```python
from build123d import *

# Parameters (mm, degrees)
F0_W     = 13
F0_H     = 6
F1_DEPTH = 17
F2_W     = 13.75
F2_H     = 6.75
F2_W_2   = 13
F2_H_2   = 6
F3_DEPTH = 0.5
F4_W     = 12.25
F4_H     = 5.25
F5_DEPTH = 16.5


with BuildPart() as f1:
    # F0 (on Top) → F1 (new body)
    with BuildSketch(Plane.XY):
        Rectangle(F0_W, F0_H)
    extrude(amount=F1_DEPTH)

    # F2 (on face) → F3 (join)
    with BuildSketch(Plane.XY.offset(17)):
        Rectangle(F2_W, F2_H)
        Rectangle(F2_W_2, F2_H_2, mode=Mode.SUBTRACT)
        Rectangle(F2_W_2, F2_H_2)
    extrude(amount=-F3_DEPTH)

    # F4 (on face) → F5 (cut, through all)
    with BuildSketch(Plane.XY.offset(17)):
        Rectangle(F4_W, F4_H)
    extrude(amount=-F5_DEPTH, mode=Mode.SUBTRACT)


solid = f1.part
```
The model under review builds one solid part; all positions refer to its coordinate system, in mm. A direction names the side the tool comes from. Coordinates: 2 decimals unless noted, no trailing zeros. Write each loop counter-clockwise with the first axis right and the second up, starting at its lowest first coordinate (ties: lowest second). Pieces come first, ordered by that corner, then holes.
1) To check wall thickness, follow probe 1 along Y at (x, z) = (2, 12.25) (3 decimals); probe 2 along X at (y, z) = (0.75, 12) (3 decimals); probe 3 along Z at (x, y) = (1.5, 1.75). State the ranges of each line that lie inside material, in increasing order.
2) The part is to be moulded in two halves that separate along Y. For faces 6 (the face through (0, -3, 8)), 7 (the face through (0, 2.625, 9)), 8 (the face through (-6.5, 0, 8)), say which applies: pulls with the +Y half, pulls with the -Y half, needs draft (parallel to the pull), parting line crosses it, or undercut.
3) Clearance check with flat-ended pins moving along their axes: pin 1 Ø3 at (x, z) = (-1, 3.5) entering from -Y; pin 2 Ø1.6 at (y, z) = (-1, 5.5) entering from +X; pin 3 Ø4 at (x, y) = (-1.5, 0.5) entering from +Z. State where each tip first meets the part, or that it passes through.
4) We need section B-B on z = 9.5. State the section outline as (x, y) points (3 decimals), then the cut area to 3 significant figures.
5) Machinability: for faces 1 (the face through (0, 0, 0)), 2 (the face through (0, 3, 8)), 3 (the face through (6.125, 0, 9)), 4 (the face through (6.5, 0, 8)), 5 (the face through (-1, -3, 17)), which of the approach directions +Z, -Z, +X, -X, +Y, -Y give a long, thin tool a straight path to every point of the face, cutting with its end or side? Answer none if there is none.
6) We need section A-A on y = -2.25. State the section outline as (x, z) points (3 decimals).
7) We need section C-C on x = -2. State the section outline as (y, z) points (3 decimals).
Answer list:
1. probe 1: y = -3 to -2.625, 2.625 to 3
1. probe 2: x = -6.5 to -6.125, 6.125 to 6.5
1. probe 3: z = 0 to 0.5
2. face 6: pulls with the -Y half
2. face 7: undercut
2. face 8: needs draft
3. pin 1: stops at y = -3
3. pin 2: stops at x = 6.5
3. pin 3: stops at z = 0.5
4. outline: (-6.5, -3) - (6.5, -3) - (6.5, 3) - (-6.5, 3) - close; hole (-6.125, -2.625) - (6.125, -2.625) - (6.125, 2.625) - (-6.125, 2.625) - close
4. area: 13.7 mm2
5. face 1: -Z, +X, -X, +Y, -Y
5. face 2: -Z, +X, -X, +Y
5. face 3: +Z
5. face 4: -Z, +X, +Y, -Y
5. face 5: +Z, +X, -X, +Y, -Y
6. outline: (-6.875, 16.5) - (-6.5, 16.5) - (-6.5, 0) - (6.5, 0) - (6.5, 16.5) - (6.875, 16.5) - (6.875, 17) - (6.125, 17) - (6.125, 0.5) - (-6.125, 0.5) - (-6.125, 17) - (-6.875, 17) - close
7. outline: (-3.375, 16.5) - (-3, 16.5) - (-3, 0) - (3, 0) - (3, 16.5) - (3.375, 16.5) - (3.375, 17) - (2.625, 17) - (2.625, 0.5) - (-2.625, 0.5) - (-2.625, 17) - (-3.375, 17) - close
